Could you check a few things on this model? Use its own coordinates, in mm. Face numbers are marked on the shaded views. A direction names the side the tool comes from. Coordinates: 2 decimals unless noted, no trailing zeros. Order: outer loops, then holes, each group sorted by start corner. A loop starts at its lowest first (then second) coordinate and runs counter-clockwise, first axis right, second up. Notation, with made-up numbers: (87, 11.25) -> (141, 11.25) arc R7 ccw to (141, 23.25) -> close; hole circle Ø4 at (48.5, 61). An arc over 180 degrees is marked (long way). Return JSON: item names as keys, results as strings. Group by question number.
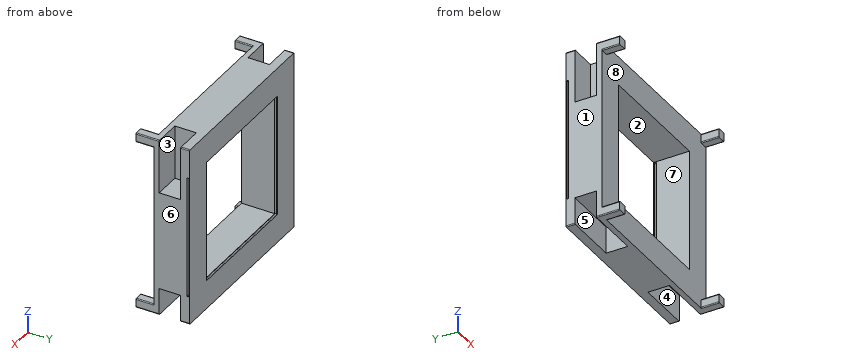
from build123d import *

# Parameters (mm, degrees)
F0_W      = 1000
F0_H      = 1000
F1_DEPTH  = 300
F2_W      = 900
F2_H      = 100
F3_DEPTH  = 1000.001
F4_W      = 100
F4_H      = 900
F5_DEPTH  = 1000.001
F6_W      = 300
F6_H      = 120
F7_DEPTH  = 150
F8_W      = 300
F8_H      = 120
F9_DEPTH  = 150
F10_W     = 120
F10_H     = 300
F11_DEPTH = 150
F12_W     = 120
F12_H     = 300
F13_DEPTH = 150
F14_R     = 5
F15_R     = 5
F16_W     = 680
F16_H     = 680
F17_DEPTH = 300.001
F18_W     = 10
F18_H     = 680
F19_DEPTH = 160.001
F20_DEPTH = 840.001


with BuildPart() as f1:
    # F0 (on Front) → F1 (new body)
    with BuildSketch(Plane.XZ):
        with Locations((450.7653813809, 448.8989327101)):
            Rectangle(F0_W, F0_H)
    extrude(amount=F1_DEPTH)

    # F2 (on face) → F3 (cut, through all)
    with BuildSketch(Plane.XY.offset(948.8989327101)):
        with Locations((450.7653813809, -250)):
            Rectangle(F2_W, F2_H)
    extrude(amount=-F3_DEPTH, mode=Mode.SUBTRACT)

    # F4 (on face) → F5 (cut, through all)
    with BuildSketch(Plane(origin=(-49.2346186191, 0, 0), x_dir=(0, -1, 0), z_dir=(-1, 0, 0))):
        with Locations((250, 448.8989327101)):
            Rectangle(F4_W, F4_H)
    extrude(amount=-F5_DEPTH, mode=Mode.SUBTRACT)

    # F6 (on face) → F7 (cut)
    with BuildSketch(Plane(origin=(0, 0, -51.1010672899), x_dir=(1, 0, 0), z_dir=(0, 0, -1))):
        with Locations((100.7653813809, 110)):
            Rectangle(F6_W, F6_H)
    extrude(amount=-F7_DEPTH, mode=Mode.SUBTRACT)

    # F8 (on face) → F9 (cut)
    with BuildSketch(Plane(origin=(0, 0, -51.1010672899), x_dir=(1, 0, 0), z_dir=(0, 0, -1))):
        with Locations((800.7653813809, 110)):
            Rectangle(F8_W, F8_H)
    extrude(amount=-F9_DEPTH, mode=Mode.SUBTRACT)

    # F10 (on face) → F11 (cut)
    with BuildSketch(Plane.YZ.offset(950.7653813809)):
        with Locations((-110, 798.8989327101)):
            Rectangle(F10_W, F10_H)
    extrude(amount=-F11_DEPTH, mode=Mode.SUBTRACT)

    # F12 (on face) → F13 (cut)
    with BuildSketch(Plane(origin=(-49.2346186191, 0, 0), x_dir=(0, -1, 0), z_dir=(-1, 0, 0))):
        with Locations((110, 798.8989327101)):
            Rectangle(F12_W, F12_H)
    extrude(amount=-F13_DEPTH, mode=Mode.SUBTRACT)

    # F14
    f14_edges = [f1.edges().sort_by_distance(p)[0] for p in [
        (950.765381, -235, -51.101067),
        (900.765381, -250, -51.101067),
        (950.765381, -250, -1.101067),
        (900.765381, -250, -1.101067),
        (-49.234619, -235, -51.101067),
        (0.765381, -250, -51.101067),
        (-49.234619, -250, -1.101067),
        (0.765381, -250, -1.101067),
        (-49.234619, -235, 948.898933),
        (0.765381, -250, 948.898933),
        (-49.234619, -250, 898.898933),
        (0.765381, -250, 898.898933),
        (950.765381, -235, 948.898933),
        (950.765381, -250, 898.898933),
        (900.765381, -250, 898.898933),
        (900.765381, -250, 948.898933),
    ]]
    fillet(f14_edges, radius=F14_R)

    # F15
    f15_edges = [f1.edges().sort_by_distance(p)[0] for p in [
        (950.765381, -25, 948.898933),
        (950.765381, -25, -51.101067),
        (-49.234619, -25, -51.101067),
        (-49.234619, -25, 948.898933),
    ]]
    fillet(f15_edges, radius=F15_R)

    # F16 (on face) → F17 (cut, through all)
    with BuildSketch(Plane(origin=(0, 0, 0), x_dir=(-1, 0, 0), z_dir=(0, 1, 0))):
        with Locations((-450.7653813809, 448.8989327101)):
            Rectangle(F16_W, F16_H)
    extrude(amount=-F17_DEPTH, mode=Mode.SUBTRACT)

    # F18 (on face) → F19 (cut, through all)
    with BuildSketch(Plane.YZ.offset(110.7653813809)):
        with Locations((-10, 445.622831583)):
            Rectangle(F18_W, F18_H)
    extrude(amount=-F19_DEPTH, mode=Mode.SUBTRACT)

    # F18 (on face) → F20 (cut, through all)
    with BuildSketch(Plane.YZ.offset(110.7653813809)):
        with Locations((-10, 445.622831583)):
            Rectangle(F18_W, F18_H)
    extrude(amount=F20_DEPTH, mode=Mode.SUBTRACT)


solid = f1.part
Q1. On a 3-axis mill with a long thin cutter (end or side, diameter ignored), from which of +Z, -Z, +X, -X, +Y, -Y can I reach the whole of each face in a straight line? I mean the marked faces 4, 5, 6, 7 and 8. Say none if no direction works.
Q2. We'd pull the mould along X, two halves only. Please class the marked faces 1, 2 and 3: pulls with the +X half, pulls with the -X half, needs draft (parallel to the pull), parting line crosses it, or undercut.
Q3. I want a section at C-C on z = 526. Please give me the cut outline in (x, y), and give its area (3 significant figures).
Q4. I want a section at B-B on y = -229.5. State how many separate pieces and enclosed holes the cut face has, and give its area (3 significant figures).
Q5. I want a section at A-A on x = 760. Please give me the cut outline in (y, z), and give its area (3 significant figures).
Q6. I need wall thicknesses on line 1 along Z through (x, y) = (737, -113); line 2 along Z through (x, y) = (532.5, -199); line 3 along X through (y, z) = (-28.5, 613.5). Which ranges of each line are inside material? Lowest first, please. Write a range as from..to.
Q7. I want a section at D-D on y = -91. Please give me the cut outline in (x, z).
Response values:
{
 "1": {"face 4": "-Z, +X", "face 5": "-Z, -X", "face 6": "+Z, -Z, +X, +Y, -Y", "face 7": "+Y, -Y", "face 8": "-Y"},
 "2": {"face 1": "pulls with the -X half", "face 2": "undercut", "face 3": "needs draft"},
 "3": {"outline": "(-49.23, -200) -> (110.77, -200) -> (110.77, -15) -> (-49.23, -15) -> close; (-49.23, -5) -> (110.77, -5) -> (110.77, 0) -> (-49.23, 0) -> close; (790.77, -200) -> (950.77, -200) -> (950.77, -15) -> (790.77, -15) -> close; (790.77, -5) -> (950.77, -5) -> (950.77, 0) -> (790.77, 0) -> close", "area": "60,800 mm²"},
 "4": {"separate pieces": "4", "enclosed holes": "0", "area": "9,910 mm²"},
 "5": {"outline": "(-200, -51.1) -> (-170, -51.1) -> (-170, 98.9) -> (-50, 98.9) -> (-50, -51.1) -> (0, -51.1) -> (0, 108.9) -> (-5, 108.9) -> (-5, 105.62) -> (-15, 105.62) -> (-15, 108.9) -> (-200, 108.9) -> close; (-200, 788.9) -> (0, 788.9) -> (0, 948.9) -> (-200, 948.9) -> close", "area": "46,000 mm²"},
 "6": {"line 1": "z = 98.9..108.9, 788.9..948.9", "line 2": "z = -51.1..108.9, 788.9..948.9", "line 3": "x = -49.23..110.77, 790.77..950.77"},
 "7": {"outline": "(-49.23, 98.9) -> (250.77, 98.9) -> (250.77, -51.1) -> (650.77, -51.1) -> (650.77, 98.9) -> (950.77, 98.9) -> (950.77, 648.9) -> (800.77, 648.9) -> (800.77, 948.9) -> (100.77, 948.9) -> (100.77, 648.9) -> (-49.23, 648.9) -> close; hole (110.77, 108.9) -> (790.77, 108.9) -> (790.77, 788.9) -> (110.77, 788.9) -> close"}
}
